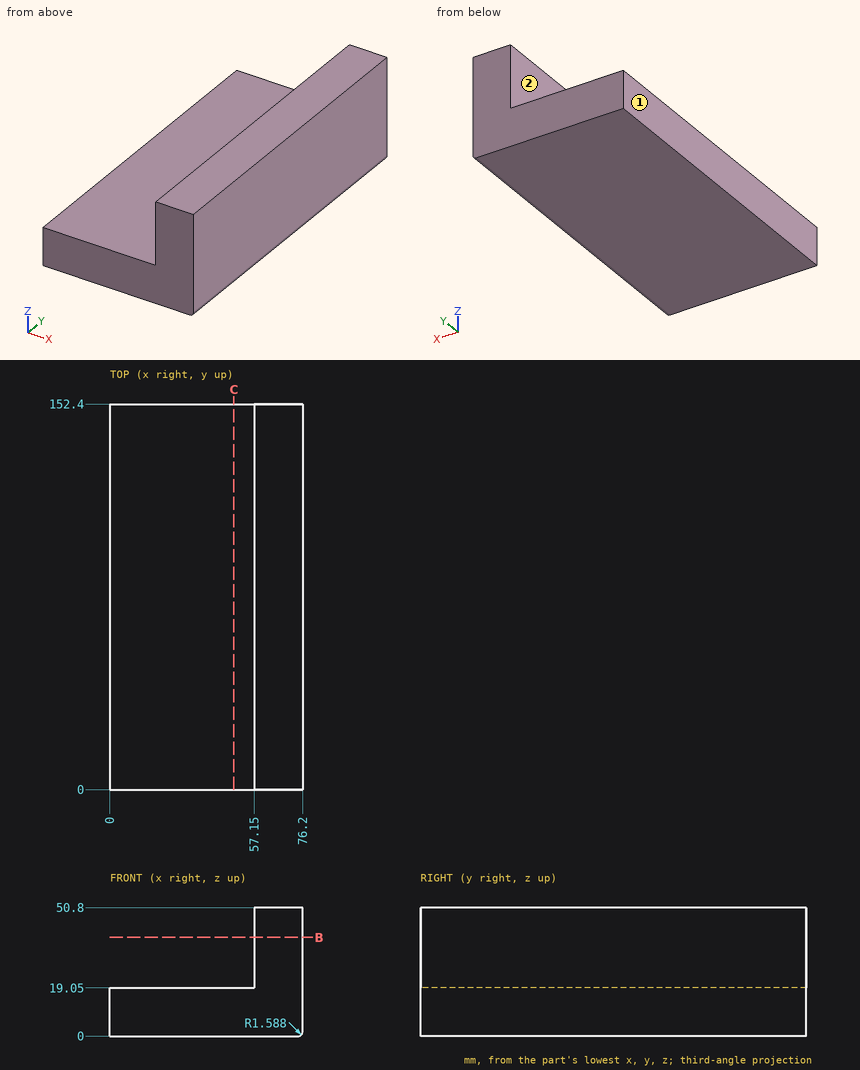
Geometry: see drawing. Coordinates: mm, zero at the bounding-box minimum. A direction names the side the tool comes from. Give positions to 0.01 mm unless a question says otherwise; leave off trailing zeros. Write each loop counter-clockwise with the first axis right and the second up, starting at its lowest first coordinate (ties: lowest second). Pieces come first, ordered by that corner, then holes. Notation, with made-up numbers: M -24.5,-20 L 24.5,-20 A19 cw 24.5,-16 Z; hole C 8.5,53.25 d1. An arc over 180 degrees is marked long. Return JSON: item names as keys, results as strings. Group by question number.
1) Cut plane B-B, the plane z = 39. Output: boundary loops of the cut face in (x, y), then the cut area to 3 significant figures.
2) Ray query, L1, parallel to Z at x = 30, y = 124.5; L2, parallel to X at y = 17.5, z = 27. Return the intervals inside material, ascending.
3) Set-up query: the marked faces 1 and 2. Return all of +Z, -Z, +X, -X, +Y, -Y with unobstructed straight access to the full face (end or side cutting, diameter ignored); none if empty.
4) First-contact query: pin 1 Ø17 at (x, y) = (36.5, 73) entering from +Z; pin 2 Ø12 at (x, z) = (49, 39) entering from +Y. Flat tips, straight axial feed; report the tip coordinate or a pass-through.
5) Cut plane C-C, the plane x = 49. Output: boundary loops of the cut face in (y, z).
Data:
{
 "1": {"outline": "M 57.15,0 L 76.2,0 L 76.2,152.4 L 57.15,152.4 Z", "area": "2,900 mm²"},
 "2": {"L1": "z = 0 to 19.05", "L2": "x = 57.15 to 76.2"},
 "3": {"face 1": "+Z, -Z, -X, +Y, -Y", "face 2": "+Z, -X, +Y, -Y"},
 "4": {"pin 1": "stops at z = 19.05", "pin 2": "passes through"},
 "5": {"outline": "M 0,0 L 152.4,0 L 152.4,19.05 L 0,19.05 Z"}
}
